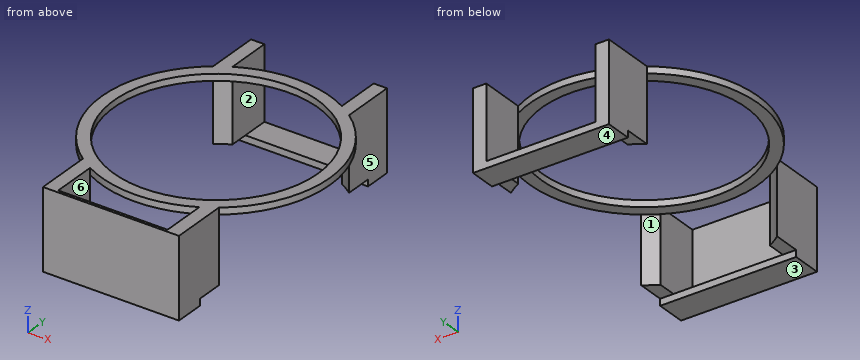
```python
from build123d import *

# Parameters (mm, degrees)
F0_R     = 42.75
F0_R_2   = 38.25
F1_DEPTH = 2.5
F3_DEPTH = 27.5
F4_W     = 51
F4_H     = 10
F5_DEPTH = 2.5
F6_W     = 51
F6_H     = 30
F7_DEPTH = 1


with BuildPart() as f1:
    # F0 (on Top) → F1 (new body)
    with BuildSketch(Plane.XY):
        Circle(F0_R)
        Circle(F0_R_2, mode=Mode.SUBTRACT)
    extrude(amount=F1_DEPTH)

    # F2 (on face) → F3 (join)
    with BuildSketch(Plane.XY.offset(2.5)):
        with BuildLine():
            Line((25.5, -54.311988), (25.5, -34.311988))
            ThreePointArc((25.5, -34.311988), (23.055661, -35.999986), (20.5, -37.514164))
            Line((20.5, -37.514164), (20.5, -54.311988))
            Line((20.5, -54.311988), (25.5, -54.311988))
        make_face()
        with BuildLine():
            ThreePointArc((-20.5, -37.514164), (-23.055661, -35.999986), (-25.5, -34.311988))
            Line((-25.5, -34.311988), (-25.5, -54.311988))
            Line((-25.5, -54.311988), (-20.5, -54.311988))
            Line((-20.5, -54.311988), (-20.5, -37.514164))
        make_face()
        with BuildLine():
            ThreePointArc((20.5, 37.514164), (23.055661, 35.999986), (25.5, 34.311988))
            Line((25.5, 34.311988), (25.5, 54.311988))
            Line((25.5, 54.311988), (20.5, 54.311988))
            Line((20.5, 54.311988), (20.5, 37.514164))
        make_face()
        with BuildLine():
            Line((-20.5, 54.311988), (-25.5, 54.311988))
            Line((-25.5, 54.311988), (-25.5, 34.311988))
            ThreePointArc((-25.5, 34.311988), (-23.055661, 35.999986), (-20.5, 37.514164))
            Line((-20.5, 37.514164), (-20.5, 54.311988))
        make_face()
    extrude(amount=-F3_DEPTH)

    # F4 (on face) → F5 (join)
    with BuildSketch(Plane(origin=(0, 0, -25), x_dir=(1, 0, 0), z_dir=(0, 0, -1))):
        with Locations((0, -49.311988)):
            Rectangle(F4_W, F4_H)
        with Locations((0, 49.311988)):
            Rectangle(F4_W, F4_H)
    extrude(amount=F5_DEPTH)

    # F6 (on face) → F7 (join)
    with BuildSketch(Plane.XZ.offset(54.311988)):
        with Locations((0, -12.5)):
            Rectangle(F6_W, F6_H)
    extrude(amount=F7_DEPTH)


solid = f1.part
```
Source: CAD feature listing. Evaluate the final solid. Frame: model axes, mm. Face numbers are marked on the shaded views. A direction names the side the tool comes from. Give positions to 0.01 mm unless a question says otherwise; leave off trailing zeros. Write each loop counter-clockwise with the first axis right and the second up, starting at its lowest first coordinate (ties: lowest second). Pieces come first, ordered by that corner, then holes.
1. Section query D-D (y = 18.5). Return the cut outline in (x, z), then the cut area to 3 significant figures.
2. Pull-direction query (X, two-part tool) for the marked faces 4, 5 and 6; classes: +X half, -X half, draft (parallel to the pull), parting line (faces both ways), or undercut.
3. Section query B-B (y = 0). Return the cut outline in (x, z).
4. Section query A-A (z = -5.5). Return the cut outline in (x, y), then the cut area to 3 significant figures.
5. Section query C-C (x = 0). Return the cut outline in (y, z), then the cut area to 4 significant figures.
6. Access query for the marked faces 1, 2 and 3. Directions: +Z, -Z, +X, -X, +Y, -Y. A direction counts if a zero-diameter tool reaches every point of the face in a straight line with its end or side. Return the directions, or none.
7. First-contact query: pin 1 (8.5 mm diameter, centred on y = 43.5, z = -15, fed in from -X); pin 2 (1.5 mm diameter, centred on x = 23, y = 39, fed in from -Z); pin 3 (5 mm diameter, centred on x = 33.5, y = 23.5, fed in from -Z); pin 4 (1.5 mm diameter, centred on y = 19, z = -1, fed in from -X) (1 decimal). Flat tips, straight axial feed; report the tip coordinate or a pass-through.
8. Material intervals for line 1 along X through (y, z) = (45.5, -7); line 2 along Y through (x, z) = (5, -18.75); line 3 along Y through (x, z) = (-14.5, 0.5), sorted ascending.
Output values:
1. outline: (-38.54, 0) - (-33.48, 0) - (-33.48, 2.5) - (-38.54, 2.5) - close; (33.48, 0) - (38.54, 0) - (38.54, 2.5) - (33.48, 2.5) - close
1. area: 25.3 mm2
2. face 4: draft
2. face 5: +X half
2. face 6: undercut
3. outline: (-42.75, 0) - (-38.25, 0) - (-38.25, 2.5) - (-42.75, 2.5) - close; (38.25, 0) - (42.75, 0) - (42.75, 2.5) - (38.25, 2.5) - close
4. outline: (-25.5, -55.31) - (25.5, -55.31) - (25.5, -34.31) arc R42.75 cw to (20.5, -37.51) - (20.5, -54.31) - (-20.5, -54.31) - (-20.5, -37.51) arc R42.75 cw to (-25.5, -34.31) - close; (-25.5, 34.31) arc R42.75 cw to (-20.5, 37.51) - (-20.5, 54.31) - (-25.5, 54.31) - close; (20.5, 37.51) arc R42.75 cw to (25.5, 34.31) - (25.5, 54.31) - (20.5, 54.31) - close
4. area: 417 mm2
5. outline: (-55.31, -27.5) - (-44.31, -27.5) - (-44.31, -25) - (-54.31, -25) - (-54.31, 2.5) - (-55.31, 2.5) - close; (-42.75, 0) - (-38.25, 0) - (-38.25, 2.5) - (-42.75, 2.5) - close; (38.25, 0) - (42.75, 0) - (42.75, 2.5) - (38.25, 2.5) - close; (44.31, -27.5) - (54.31, -27.5) - (54.31, -25) - (44.31, -25) - close
5. area: 102.5 mm2
6. face 1: -Z
6. face 2: +Z, +Y
6. face 3: -Z, +X, -X, +Y, -Y
7. pin 1: stops at x = -25.5
7. pin 2: stops at z = -25
7. pin 3: stops at z = 0
7. pin 4: passes through
8. line 1: x = -25.5 to -20.5, 20.5 to 25.5
8. line 2: y = -55.31 to -54.31
8. line 3: y = -55.31 to -54.31, -40.22 to -35.4, 35.4 to 40.22
